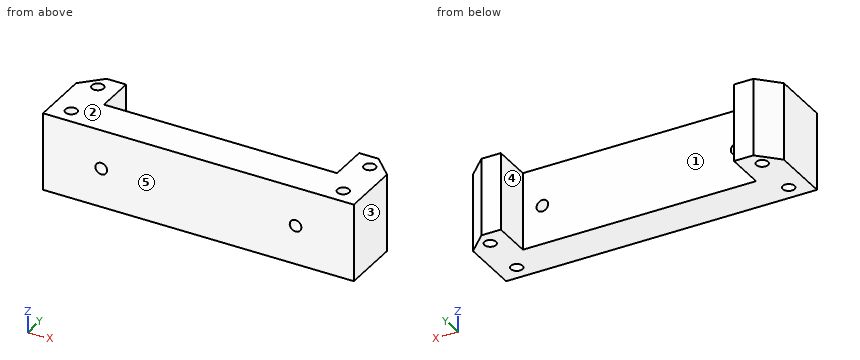
from build123d import *

# Parameters (mm, degrees)
SKETCH_1_W          = 80
SKETCH_1_H          = 20
EXTRUDE_1_DEPTH     = 20
SKETCH_2_W          = 60
SKETCH_2_H          = 20
CUT_EXTRUDE_1_DEPTH = 10
SKETCH_3_R          = 1.5
CUT_EXTRUDE_2_DEPTH = 43.426406871
CHAMFER_1_SIZE      = 5
SKETCH_4_R          = 1.5
CUT_EXTRUDE_3_DEPTH = 49.989794856


with BuildPart() as part:
    # 草图1 → 凸台-拉伸1 (new body)
    with BuildSketch(Plane(origin=(0, 0, 0), x_dir=(1, 0, 0), z_dir=(0, 1, 0))):
        Rectangle(SKETCH_1_W, SKETCH_1_H)
    extrude(amount=EXTRUDE_1_DEPTH)

    # 草图2 → 切除-拉伸1 (cut)
    with BuildSketch(Plane(origin=(0, 20, 0), x_dir=(1, 0, 0), z_dir=(0, 1, 0))):
        Rectangle(SKETCH_2_W, SKETCH_2_H)
    extrude(amount=-CUT_EXTRUDE_1_DEPTH, mode=Mode.SUBTRACT)

    # 草图3 → 切除-拉伸2 (cut, through all)
    with BuildSketch(Plane(origin=(0, 10, 0), x_dir=(1, 0, 0), z_dir=(0, 1, 0))):
        with Locations(Location((-25, 0, 0), (0, 0, 270))):
            Circle(SKETCH_3_R)
        with Locations(Location((25, 0, 0), (0, 0, 90))):
            Circle(SKETCH_3_R)
    extrude(amount=-CUT_EXTRUDE_2_DEPTH, mode=Mode.SUBTRACT)

    # 倒角1
    chamfer_1_edges = [part.edges().sort_by_distance(p)[0] for p in [
        (-40, 20, 0),
        (40, 20, 0),
    ]]
    chamfer(chamfer_1_edges, length=CHAMFER_1_SIZE)

    # 草图4 → 切除-拉伸3 (cut, through all)
    with BuildSketch(Plane.XY.offset(10)):
        with Locations((-35, 16)):
            Circle(SKETCH_4_R)
        with Locations(Location((-35, 4, 0), (0, 0, 180))):
            Circle(SKETCH_4_R)
        with Locations((35, 4)):
            Circle(SKETCH_4_R)
        with Locations(Location((35, 16, 0), (0, 0, 180))):
            Circle(SKETCH_4_R)
    extrude(amount=-CUT_EXTRUDE_3_DEPTH, mode=Mode.SUBTRACT)


solid = part.part
CAD build for the part. Positions are in the model's coordinates, mm. Face numbers are marked on the shaded views. A direction names the side the tool comes from. Give positions to 0.01 mm unless a question says otherwise; leave off trailing zeros. Loops run counter-clockwise (first coordinate to the right, second up) from the corner with the lowest first, then second, coordinate; pieces in that order, holes last. Notation, with made-up numbers: M 37.25,11 L 61.25,11 A24 ccw 61.25,24 Z; hole C 86,51 d3. An arc over 180 degrees is marked long. Answer in a Markdown table with one row per item. Add a question column.
Item 1: Mould opens along X. For the marked faces 3, 4 and 5 say: +X half, -X half, draft (parallel to the pull), parting line (faces both ways), or undercut.
Item 2: Probe probe 1 along X at (y, z) = (13.75, 4.5); probe 2 along X at (y, z) = (3.5, 8.25); probe 3 along X at (y, z) = (16.5, 7.25). List the from-to ranges inside material, lowest first.
Item 3: Band-saw the part on C-C on x = -25. Give the cut face in (y, z).
Item 4: Tool access for the marked faces 1 and 2: list every direction of +Z, -Z, +X, -X, +Y, -Y with a clear straight run to the whole face (end or side of a thin tool).
Item 5: Band-saw the part on D-D on z = -4.75. Give the cut face in (x, y), then the cut area to 3 significant figures.
Item 6: Band-saw the part on B-B on y = 18.5. Give the cut face in (x, z).
Item 7: Drop flat-ended pins along their axis: P1, Ø6, axis at x = 11, z = -4.5, coming from the +Y side; P2, Ø2.5, axis at x = 35, y = 4, coming from the +Z side. Give the stop position or say it passes through.
Item 8: Band-saw the part on A-A on y = 4. Give the cut face in (x, z), then the cut area to 3 significant figures.
Reply:
| question | item | result |
|---|---|---|
| 1 | face 3 | +X half |
| 1 | face 4 | undercut |
| 1 | face 5 | draft |
| 2 | probe 1 | x = -40 to -30, 30 to 40 |
| 2 | probe 2 | x = -40 to -36.41, -33.59 to 33.59, 36.41 to 40 |
| 2 | probe 3 | x = -38.5 to -36.41, -33.59 to -30, 30 to 33.59, 36.41 to 38.5 |
| 3 | outline | M 0,-10 L 10,-10 L 10,-1.5 L 0,-1.5 Z; M 0,1.5 L 10,1.5 L 10,10 L 0,10 Z |
| 4 | face 1 | +Z, -Z, +Y |
| 4 | face 2 | +Z, +X, -X, +Y, -Y |
| 5 | outline | M -40,0 L 40,0 L 40,15 L 35,20 L 30,20 L 30,10 L -30,10 L -30,20 L -35,20 L -40,15 Z; hole C -35,4 d3; hole C -35,16 d3; hole C 35,4 d3; hole C 35,16 d3 |
| 5 | area | 947 mm^2 |
| 6 | outline | M -36.5,-10 L -30,-10 L -30,10 L -36.5,10 Z; M 30,-10 L 36.5,-10 L 36.5,10 L 30,10 Z |
| 7 | P1 | stops at y = 10 |
| 7 | P2 | passes through |
| 8 | outline | M -40,-10 L -36.5,-10 L -36.5,10 L -40,10 Z; M -33.5,-10 L 33.5,-10 L 33.5,10 L -33.5,10 Z; M 36.5,-10 L 40,-10 L 40,10 L 36.5,10 Z; hole C -25,0 d3; hole C 25,0 d3 |
| 8 | area | 1,470 mm^2 |
